from build123d import *

# Parameters (mm, degrees)
F0_W     = 25
F0_H     = 25
F1_DEPTH = 25
F2_R     = 5
F3_T     = -3


# Not quite as in the source:
# - a shell that OpenCascade refuses in one call is made with other operations: the cavity is built on its own and cut out


with BuildPart() as f1:
    # F0 (on Front) → F1 (new body)
    with BuildSketch(Plane.XZ):
        with Locations((12.5, 12.5)):
            Rectangle(F0_W, F0_H)
    extrude(amount=F1_DEPTH)

    # F2
    f2_edges = [f1.edges().sort_by_distance(p)[0] for p in [
        (12.5, 0, 0),
        (25, -12.5, 0),
        (25, -12.5, 25),
        (12.5, 0, 25),
        (12.5, -25, 25),
        (0, -12.5, 25),
        (12.5, -25, 0),
        (0, -25, 12.5),
        (0, 0, 12.5),
        (0, -12.5, 0),
    ]]
    fillet(f2_edges, radius=F2_R)

    # F3: a shell. OpenCascade refuses it in one call, so the cavity is built on its own and cut out:
    # the body offset inwards by the wall thickness, plus a prism from it out through each open face.
    f3_core = offset(f1.part, amount=F3_T, mode=Mode.PRIVATE)
    f3_exits = [f3_core.faces().sort_by_distance(p)[0] for p in [
        (12.5, -12.5, 3),
    ]]
    add(f3_core, mode=Mode.SUBTRACT)
    extrude(f3_exits, amount=-F3_T, mode=Mode.SUBTRACT)


solid = f1.part
Geometry check sheet. Reference: the model listing, model coordinates, mm. A direction names the side the tool comes from. Round coordinates to 2 decimals unless told otherwise and drop trailing zeros. Order: outer loops, then holes, each group sorted by start corner. A loop starts at its lowest first (then second) coordinate and runs counter-clockwise, first axis right, second up. Notation, with made-up numbers: (68, 20.5) -> (95, 20.5) arc R14 cw to (95, 29.5) -> close; hole circle Ø2 at (64.5, 76). An arc over 180 degrees is marked (long way). Use one line per item in the form item = value.
1. Cross-section at A-A, the plane z = 8.5. Enter the section's corners in (x, y), plus the area to 3 significant figures.
Working result:
outline = (0, -20) arc R5 ccw to (5, -25) -> (25, -25) -> (25, 0) -> (5, 0) arc R5 ccw to (0, -5) -> close; hole (3, -20) arc R2 ccw to (5, -22) -> (22, -22) -> (22, -3) -> (5, -3) arc R2 ccw to (3, -5) -> close
area = 255 mm^2
2. Cross-section at C-C, the plane y = -9.25. Enter the section's corners in (x, z).
Working result:
outline = (0, 5) arc R5 ccw to (5, 0) -> (5, 3) arc R2 cw to (3, 5) -> (3, 20) arc R2 cw to (5, 22) -> (20, 22) arc R2 cw to (22, 20) -> (22, 5) arc R2 cw to (20, 3) -> (20, 0) arc R5 ccw to (25, 5) -> (25, 20) arc R5 ccw to (20, 25) -> (5, 25) arc R5 ccw to (0, 20) -> close
3. Cross-section at B-B, the plane x = 5.5. Enter the section's corners in (y, z).
Working result:
outline = (-25, 5) arc R5 ccw to (-20, 0) -> (-20, 3) arc R2 cw to (-22, 5) -> (-22, 20) arc R2 cw to (-20, 22) -> (-5, 22) arc R2 cw to (-3, 20) -> (-3, 5) arc R2 cw to (-5, 3) -> (-5, 0) arc R5 ccw to (0, 5) -> (0, 20) arc R5 ccw to (-5, 25) -> (-20, 25) arc R5 ccw to (-25, 20) -> close
4. Scan lines: line 1 along X through (y, z) = (-16.25, 5.75); line 2 along Y through (x, z) = (16.5, 11); line 3 along Z through (x, y) = (20.5, -9.25). Record each from-to range of solid material in increasing order. Write a range as from..to.
Working result:
line_1 = 0..3, 22..25
line_2 = -25..-22, -3..0
line_3 = 0.03..3.06, 21.94..24.97
5. Go/stop test with flat-tipped pins: pin 1 (0.9 mm diameter, centred on x = 14.5, z = 1, fed in from +Y); pin 2 (2.5 mm diameter, centred on y = -14.5, z = 1.5, fed in from -X); pin 3 (3 mm diameter, centred on x = 20.5, y = -22, fed in from -Z). Record where each tip stops, or that it passes through.
Working result:
pin_1 = -1.48
pin_2 = 0.53
pin_3 = 0.03
6. Set-up check for faces 1 (the face through (5, -12, 2)), 2 (the face through (1, -13, 2)), 3 (the face through (13, -3, 13)): record each of +Z, -Z, +X, -X, +Y, -Y from which the full face is reachable in a straight line by a thin tool's end or side.
Working result:
face_1 = -Z
face_2 = -Z, -X, +Y, -Y
face_3 = none
7. Cross-section at D-D, the plane y = -21. Enter the section's corners in (x, z).
Working result:
outline = (0.1, 5) arc R4.9 ccw to (5, 0.1) -> (21, 0.1) arc R5 ccw to (25, 5) -> (25, 20) arc R5 ccw to (21, 24.9) -> (5, 24.9) arc R4.9 ccw to (0.1, 20) -> close; hole (3.27, 5) arc R1.73 ccw to (5, 3.27) -> (21, 3.27) arc R2 ccw to (22, 5) -> (22, 20) arc R2 ccw to (21, 21.73) -> (5, 21.73) arc R1.73 ccw to (3.27, 20) -> close
8. Mould release check, pull along Z, two halves, no side actions. Record for faces 4 (the face through (21.43, -12.63, 21.4)), 5 (the face through (15, -23, 24)), 6 (the face through (15, -23, 1)): pulls with the +Z half, pulls with the -Z half, needs draft (parallel to the pull), parting line crosses it, or undercut.
Working result:
face_4 = undercut
face_5 = pulls with the +Z half
face_6 = pulls with the -Z half
